Build history of the part. All positions in model axes, mm. A direction names the side the tool comes from. Give positions to 0.01 mm unless a question says otherwise; leave off trailing zeros. Loops run counter-clockwise (first coordinate to the right, second up) from the corner with the lowest first, then second, coordinate; pieces in that order, holes last. Notation, with made-up numbers: (51, 18) -> (61, 18) arc R9 ccw to (61, 22) -> close; hole circle Ø8 at (76, -21). An arc over 180 degrees is marked (long way). Answer as a JSON object with one key per item and string values. Group by question number.
Q1. Tool access for faces 1 (the flat face through (0, 35, 10)), 2 (the flat face through (-3, 27.8, 10)), 3 (the cylindrical face through (27.62, 43.7, 10.33)), 4 (the flat face through (43, 27.8, 10)): list every direction of +Z, -Z, +X, -X, +Y, -Y with a clear straight run to the whole face (end or side of a thin tool).
Q2. Wall check: probe 1 along Z at (x, y) = (-4.75, 29.7); probe 2 along Z at (x, y) = (44, 28); probe 3 along X at (y, z) = (9, 8). Give the ranges that are in metal, low to high. Write a range as from..to.
Q3. Drop flat-ended pins along their axis: pin 1 (3 mm diameter, centred on x = 44.75, z = 5, fed in from +Y); pin 2 (8 mm diameter, centred on y = 38, z = 15, fed in from +X); pin 3 (6 mm diameter, centred on x = 44.75, z = 15, fed in from -Y); pin 4 (11 mm diameter, centred on y = 37.5, z = 15, fed in from -X). Give the stop position or say it passes through.
Q4. Band-saw the part on A-A, the plane x = 44.75. Write the cut outline in (y, z).
Q5. Band-saw the part on C-C, the plane x = 30.1. Write the cut outline in (y, z).
Q6. Two-plate mould, pull along Z, no slides. Class faces 5 (the flat face through (47.25, 29, 10)), 6 (the flat face through (20, 20, 0)), 7 (the cylindrical face through (-2.15, 29.12, 15.1)): pulls with the +Z half, pulls with the -Z half, needs draft (parallel to the pull), parting line crosses it, or undercut.
Q7. Band-saw the part on D-D, the plane y = 26. Write the cut outline in (x, z).
Q8. Band-saw the part on B-B, the plane z = 10. Write the cut outline in (x, y), plus the area to 3 significant figures.
from build123d import *

# Parameters (mm, degrees)
SKETCH1_W           = 40
SKETCH1_H           = 20
BOSS_EXTRUDE1_DEPTH = 40.5
SKETCH2_R           = 2.5
BOSS_EXTRUDE2_DEPTH = 6.5
SKETCH3_W           = 20
SKETCH3_H           = 2.6
BOSS_EXTRUDE3_DEPTH = 7.25
SKETCH4_W           = 20
SKETCH4_H           = 2.6
BOSS_EXTRUDE4_DEPTH = 7.25
SKETCH5_R           = 2.6
CUT_EXTRUDE5_DEPTH  = 7.25


with BuildPart() as part:
    # Sketch1 → Boss-Extrude1 (new body)
    with BuildSketch(Plane(origin=(0, 0, 0), x_dir=(1, 0, 0), z_dir=(0, 1, 0))):
        with Locations((20, -10)):
            Rectangle(SKETCH1_W, SKETCH1_H)
    extrude(amount=BOSS_EXTRUDE1_DEPTH)

    # Sketch2 → Boss-Extrude2 (add)
    with BuildSketch(Plane(origin=(0, 40.5, 0), x_dir=(1, 0, 0), z_dir=(0, 1, 0))):
        with Locations(Location((30.1, -10, 0), (0, 0, 90))):
            Circle(SKETCH2_R)
    extrude(amount=BOSS_EXTRUDE2_DEPTH)

    # Sketch3 → Boss-Extrude3 (add)
    with BuildSketch(Plane.ZY):
        with Locations((10, 29.1)):
            Rectangle(SKETCH3_W, SKETCH3_H)
    extrude(amount=BOSS_EXTRUDE3_DEPTH)

    # Sketch4 → Boss-Extrude4 (add)
    with BuildSketch(Plane(origin=(40, 0, 0), x_dir=(0, 0, -1), z_dir=(1, 0, 0))):
        with Locations((-10, 29.1)):
            Rectangle(SKETCH4_W, SKETCH4_H)
    extrude(amount=BOSS_EXTRUDE4_DEPTH)

    # Sketch5 → Cut-Extrude5 (cut)
    with BuildSketch(Plane(origin=(0, 30.4, 0), x_dir=(1, 0, 0), z_dir=(0, 1, 0))):
        with Locations((44.75, -5)):
            Circle(SKETCH5_R)
        with Locations((44.75, -15)):
            Circle(SKETCH5_R)
        with Locations((-4.75, -15)):
            Circle(SKETCH5_R)
        with Locations((-4.75, -5)):
            Circle(SKETCH5_R)
    extrude(amount=-CUT_EXTRUDE5_DEPTH, mode=Mode.SUBTRACT)


solid = part.part
Worked answers:
{
 "1": {"face 1": "+Z, -Z, -X, +Y", "face 2": "+Z, -Z, -X, -Y", "face 3": "+Y", "face 4": "+Z, -Z, +X, -Y"},
 "2": {"probe 1": "0..2.4, 7.6..12.4, 17.6..20", "probe 2": "0..2.51, 7.49..12.51, 17.49..20", "probe 3": "0..40"},
 "3": {"pin 1": "through", "pin 2": "x = 40", "pin 3": "y = 27.8", "pin 4": "x = 0"},
 "4": {"outline": "(27.8, 0) -> (30.4, 0) -> (30.4, 2.4) -> (27.8, 2.4) -> close; (27.8, 7.6) -> (30.4, 7.6) -> (30.4, 12.4) -> (27.8, 12.4) -> close; (27.8, 17.6) -> (30.4, 17.6) -> (30.4, 20) -> (27.8, 20) -> close"},
 "5": {"outline": "(0, 0) -> (40.5, 0) -> (40.5, 7.5) -> (47, 7.5) -> (47, 12.5) -> (40.5, 12.5) -> (40.5, 20) -> (0, 20) -> close"},
 "6": {"face 5": "needs draft", "face 6": "pulls with the -Z half", "face 7": "undercut"},
 "7": {"outline": "(0, 0) -> (40, 0) -> (40, 20) -> (0, 20) -> close"},
 "8": {"outline": "(-7.25, 27.8) -> (0, 27.8) -> (0, 0) -> (40, 0) -> (40, 27.8) -> (47.25, 27.8) -> (47.25, 30.4) -> (40, 30.4) -> (40, 40.5) -> (32.6, 40.5) -> (32.6, 47) -> (27.6, 47) -> (27.6, 40.5) -> (0, 40.5) -> (0, 30.4) -> (-7.25, 30.4) -> close", "area": "1,690 mm2"}
}
